Autodesk Inventor part; units mm, degrees
ref_plane "YZ Plane" through (0, 0, 0) normal (1, 0, 0) x (0, 1, 0)
ref_plane "XZ Plane" through (0, 0, 0) normal (0, 1, 0) x (-1, 0, 0)
ref_plane "XY Plane" through (0, 0, 0) normal (0, 0, 1) x (1, 0, 0)
sketch "Sketch1" plane through (0, 0, 0) normal (0, 0, 1) x (1, 0, 0)
  line L0 (-37.0102, 0) -> (-37.0102, 16.1)
  line L1 (-37.0102, 16.1) -> (6.7898, 16.1)
  line L2 (6.7898, 16.1) -> (6.7898, 17.7)
  line L3 (6.7898, 17.7) -> (31.0898, 17.7)
  line L4 (31.0898, 17.7) -> (31.0898, 0)
  line L5 (31.0898, 0) -> (-37.0102, 0)
  line L6 (-42.8743, 0) -> (48.8507, 0) construction
  line L7 (0, 23.2775) -> (0, -29.7437) construction
  point P0 (0, 0)
  dimension "d0" = 16.1
  dimension "d1" = 68.1
  dimension "d2" = 24.3
  dimension "d3" = 17.7
revolve "Revolution1" add sketch "Sketch1" angle 360 about axis through (-42.8743, 0, 0) along (1, 0, 0)
sketch "Sketch2" plane through (31.0898, 0, 0) normal (1, 0, 0) x (0, 0, -1)
  point P0 (0, 0)
  point P1 (0, 8.73)
  dimension "d5" = 8.73
sketch "Sketch3" plane through (0, 0, 0) normal (0, 0, 1) x (1, 0, 0)
  line L0 (31.0898, 8.73) -> (43.5898, 8.73)
  line L1 (43.5898, 8.73) -> (43.5898, 11.23)
  line L2 (43.5898, 11.23) -> (32.5898, 11.23)
  line L3 (32.5898, 11.23) -> (32.5898, 14.73)
  line L4 (32.5898, 14.73) -> (31.0898, 14.73)
  line L5 (31.0898, 14.73) -> (31.0898, 8.73)
  line L6 (24.3312, 8.73) -> (72.9935, 8.73) construction
  line L7 (6.7898, -17.7) -> (6.7898, 17.7) construction
  point P0 (0, 0)
  dimension "d6" = 6
  dimension "d8" = 2.5
  dimension "d9" = 1.5
  dimension "d10" = 12.5
revolve "Revolution2" add sketch "Sketch3" angle 360 about axis through (24.3312, 8.73, 0) along (1, 0, 0)
sketch "Sketch4" plane through (0, 0, 0) normal (0, 0, 1) x (1, 0, 0)
  line L0 (32.5898, 6.23) -> (43.5898, 6.23)
  line L1 (43.5898, 6.23) -> (34.0898, 6.23)
  line L2 (34.0898, 6.23) -> (34.0898, 7.23)
  line L3 (34.0898, 7.23) -> (43.5898, 7.23)
  line L4 (43.5898, 7.23) -> (43.5898, 6.23)
  point P0 (0, 0)
  dimension "d12" = 1
  dimension "d13" = 9.5
extrude "Extrusion1" cut sketch "Sketch4" along normal mid plane 10
sketch "Sketch5" plane through (31.0898, 0, 0) normal (1, 0, 0) x (0, 0, -1)
  line L0 (0, -24.78) -> (0, 24.78)
  line L1 (-24.78, 0) -> (24.78, 0)
  point P0 (0, 0)
  point P1 (-10.25, 8.73)
  point P2 (10.25, 8.73)
  point P3 (0, -13.37)
  dimension "d16" = 20.5
  dimension "d17" = 8.73
  dimension "d18" = 22.1
hole "Hole1" at (31.0898, 8.73, 10.25) at (31.0898, 8.73, -10.25) at (31.0898, -13.37, 0) direction (-1, 0, 0) diameter 2.459 depth 4.5
sketch "Sketch6" plane through (-37.0102, 0, 0) normal (-1, 0, 0) x (0, 0, 1)
  line L0 (0, 24.78) -> (0, -24.78)
  line L1 (-24.78, 0) -> (24.78, 0)
  line L2 (-1.4, 11.75) -> (1.4, 11.75)
  line L3 (1.4, 11.75) -> (1.4, 11.25)
  line L4 (1.4, 11.25) -> (-1.4, 11.25)
  line L5 (-1.4, 11.25) -> (-1.4, 11.75)
  line L6 (-1.4, -11.75) -> (1.4, -11.75)
  line L7 (1.4, -11.75) -> (1.4, -11.25)
  line L8 (1.4, -11.25) -> (-1.4, -11.25)
  line L9 (-1.4, -11.25) -> (-1.4, -11.75)
  point P0 (0, 0)
  point P1 (0, 11.25)
  point P2 (0, -11.25)
  dimension "d26" = 2.8
  dimension "d27" = 0.5
  dimension "d28" = 11.25
extrude "Extrusion2" add sketch "Sketch6" along normal blind 9.5
properties material "Thermoplastic Resin"
Build history of the part. All positions in model axes, mm. A direction names the side the tool comes from. Round coordinates to 2 decimals unless told otherwise and drop trailing zeros. Write each loop counter-clockwise with the first axis right and the second up, starting at its lowest first coordinate (ties: lowest second). Pieces come first, ordered by that corner, then holes. Notation, with made-up numbers: (41.5, 32) - (56.5, 32) arc R10 ccw to (56.5, 42) - close; hole circle Ø3 at (49.25, 47). An arc over 180 degrees is marked (long way). One line per question, with ' | ' between items.
1. Mould opens along Y. For faces 1 (the face through (31.83, 14.27, 2.3)), 2 (the face through (28.81, -14.59, 0.16)), 3 (the face through (-42, -11.75, 0)) say: released by +Y, released by -Y, zero draft, split by the parting line, or undercut.
Results are:
face 1: split by the parting line | face 2: undercut | face 3: released by -Y
2. Band-saw the part on B-B, the plane y = 0. Write the cut outline in (x, z), and give its area (3 significant figures).
Results are:
outline: (-37.01, -16.1) - (6.79, -16.1) - (6.79, -17.7) - (31.09, -17.7) - (31.09, 17.7) - (6.79, 17.7) - (6.79, 16.1) - (-37.01, 16.1) - close | area: 2,270 mm^2
3. Drop flat-ended pins along their axis: pin 1 Ø2 at (x, z) = (-41, -0.5) entering from -Y; pin 2 Ø1 at (x, y) = (10, 6) entering from +Z; pin 3 Ø3 at (y, z) = (-10.5, 2) entering from +X. Give the stop position or say it passes through.
Results are:
pin 1: y = -11.75 | pin 2: z = 16.82 | pin 3: x = 31.09
4. Drill centre lines: line 1 along Z through (x, y) = (28.2, 8.73); line 2 along X through (y, z) = (2.5, 5); line 3 along Z through (x, y) = (17, -0.5). Where is each one in solid material? Low to high. Write a range as from..to.
Results are:
line 1: -15.4..-11.48, -9.02..9.02, 11.48..15.4 | line 2: -37.01..31.09 | line 3: -17.69..17.69
5. Band-saw the part on C-C, the plane x = -24. Write the cut outline in (y, z), and give its area (3 significant figures).
Results are:
outline: circle Ø32.2 at (0, 0) | area: 814 mm^2
6. Band-saw the part on D-D, the plane y = -9.5. Write the cut outline in (x, z).
Results are:
outline: (-37.01, -13) - (6.79, -13) - (6.79, -14.93) - (31.09, -14.93) - (31.09, 14.93) - (6.79, 14.93) - (6.79, 13) - (-37.01, 13) - close
7. Tool access for faces 4 (the face through (19.11, 16.88, 5.32)), 5 (the face through (-42, -11.25, 0)), 6 (the face through (-14.804, 15.357, 4.836)), 7 (the face through (26.59, 9, 10)), 8 (the face through (-42, 11.75, 0)): list every direction of +Z, -Z, +X, -X, +Y, -Y with a clear straight run to the whole face (end or side of a thin tool).
Results are:
face 4: +X, -X | face 5: +Z, -Z, -X | face 6: -X | face 7: +X | face 8: +Z, -Z, -X, +Y
